Read the model definition and answer for the solid it produces. Units are mm, in the model's axes. A direction names the side the tool comes from. Coordinates: 2 decimals unless noted, no trailing zeros. Write each loop counter-clockwise with the first axis right and the second up, starting at its lowest first coordinate (ties: lowest second). Pieces come first, ordered by that corner, then holes. Notation, with made-up numbers: (78, -33.75) -> (110, -33.75) arc R23 cw to (110, -4.75) -> close; hole circle Ø9 at (45.5, -6). An arc over 180 degrees is marked (long way). Return JSON: item names as keys, results as strings.
from build123d import *

# Parameters (mm, degrees)
SKETCH1_W           = 5.23
SKETCH1_H           = 5.23
BOSS_EXTRUDE1_DEPTH = 14
FILLET1_R           = 1
FILLET2_R           = 1


with BuildPart() as part:
    # Sketch1 → Boss-Extrude1 (new body)
    with BuildSketch(Plane.XY):
        with BuildLine():
            Line((-6, 0), (-6, 10))
            ThreePointArc((-6, 10), (0, 16), (6, 10))
            Line((6, 10), (6, 0))
            ThreePointArc((6, 0), (0, -6), (-6, 0))
        make_face()
        with Locations((0, 7.9)):
            Rectangle(SKETCH1_W, SKETCH1_H, mode=Mode.SUBTRACT)
    extrude(amount=BOSS_EXTRUDE1_DEPTH)

    # Fillet1
    fillet1_edges = [part.edges().sort_by_distance(p)[0] for p in [
        (2.615, 7.9, 14),
        (0, 10.515, 14),
        (-2.615, 7.9, 14),
        (0, 5.285, 14),
    ]]
    fillet(fillet1_edges, radius=FILLET1_R)

    # Fillet2
    fillet2_edges = [part.edges().sort_by_distance(p)[0] for p in [
        (2.615, 7.9, 0),
        (0, 10.515, 0),
        (-2.615, 7.9, 0),
        (0, 5.285, 0),
    ]]
    fillet(fillet2_edges, radius=FILLET2_R)


solid = part.part
1. Consider L1, parallel to X at y = 7.5, z = 3.25 (3 decimals); L2, parallel to Y at x = -1.5, z = 9 (3 decimals); L3, parallel to Y at x = -2.5, z = 9.25 (3 decimals). Determine where each line is inside the solid, lowest interval first.
Taken from the geometry:
{"L1": "x = -6 to -2.615, 2.615 to 6", "L2": "y = -5.809 to 5.285, 10.515 to 15.809", "L3": "y = -5.454 to 5.285, 10.515 to 15.454"}
2. The part is cut by section C-C (z = 3.75). Determine the outline of the cut face in (x, y) (3 decimals).
Taken from the geometry:
{"outline": "(-6, 0) arc R6 ccw to (6, 0) -> (6, 10) arc R6 ccw to (-6, 10) -> close; hole (-2.615, 5.285) -> (2.615, 5.285) -> (2.615, 10.515) -> (-2.615, 10.515) -> close"}
3. The part is cut by section D-D (y = 11). Determine the outline of the cut face in (x, z) (3 decimals).
Taken from the geometry:
{"outline": "(-5.916, 0) -> (-3.615, 0) arc R1 ccw to (-3.1, 0.143) -> (3.1, 0.143) arc R1 ccw to (3.615, 0) -> (5.916, 0) -> (5.916, 14) -> (3.615, 14) arc R1 ccw to (3.1, 13.857) -> (-3.1, 13.857) arc R1 ccw to (-3.615, 14) -> (-5.916, 14) -> close"}
4. For a pull along Y with two mould halves and no side action, classify faces 1 (the face through (2.9, 8, 0.3)), 2 (the face through (-6, 5, 7)), 3 (the face through (0, -6, 7)) as +Y half, -Y half, draft (parallel to the pull), parting line (faces both ways), or undercut.
Taken from the geometry:
{"face 1": "undercut", "face 2": "draft", "face 3": "-Y half"}
5. The part is cut by section A-A (y = 7.75). Determine the outline of the cut face in (x, z) (3 decimals), then the cut area to 3 significant figures.
Taken from the geometry:
{"outline": "(-6, 0) -> (-3.615, 0) arc R1 ccw to (-2.615, 1) -> (-2.615, 13) arc R1 ccw to (-3.615, 14) -> (-6, 14) -> close; (2.615, 1) arc R1 ccw to (3.615, 0) -> (6, 0) -> (6, 14) -> (3.615, 14) arc R1 ccw to (2.615, 13) -> close", "area": "93.9 mm2"}
6. Flat-ended cylindrical pins translate along their axes: pin 1 Ø1.5 at (x, z) = (-4, 8) entering from -Y; pin 2 Ø2 at (y, z) = (12.5, 8) entering from +X; pin 3 Ø3 at (y, z) = (12, 6) entering from -X. Find the tip coordinate at first contact, or state that the pin passes through.
Taken from the geometry:
{"pin 1": "stops at y = -5.04", "pin 2": "stops at x = 5.81", "pin 3": "stops at x = -5.98"}
7. The part is cut by section B-B (x = 0). Determine the outline of the cut face in (y, z) (3 decimals), then the cut area to 3 significant figures.
Taken from the geometry:
{"outline": "(-6, 0) -> (4.285, 0) arc R1 ccw to (5.285, 1) -> (5.285, 13) arc R1 ccw to (4.285, 14) -> (-6, 14) -> close; (10.515, 1) arc R1 ccw to (11.515, 0) -> (16, 0) -> (16, 14) -> (11.515, 14) arc R1 ccw to (10.515, 13) -> close", "area": "234 mm2"}
8. A tool of negligible diameter and unlimited length cuts with its end or side. For faces 4 (the face through (-2.9, 8, 13.7)), 5 (the face through (0, 3, 14)), 6 (the face through (0, 16, 7)), 7 (the face through (0.1, 5, 0.3)), 8 (the face through (-2.615, 8, 7)), from which of +Z, -Z, +X, -X, +Y, -Y can it reach the whole face along a straight path? Write none if from no direction.
Taken from the geometry:
{"face 4": "+Z", "face 5": "+Z, +X, -X, +Y, -Y", "face 6": "+Z, -Z, +Y", "face 7": "-Z", "face 8": "+Z, -Z"}
